Autodesk Inventor part; units mm, degrees
ref_plane "Work Plane1" through (1.525, 0, 0) normal (0, 0, 1) x (1, 0, 0)
ref_plane "YZ Plane" through (0, 0, 0) normal (1, 0, 0) x (0, 1, 0)
ref_plane "XZ Plane" through (0, 0, 0) normal (0, 1, 0) x (-1, 0, 0)
sketch "Sketch1" plane through (0, 0, 0) normal (0, 0, 1) x (1, 0, 0)
  line L0 (0, 4) -> (0, 2.5)
  line L1 (2.4, 2.5) -> (10, 2.5)
  line L2 (10, 2.5) -> (10, 0)
  line L3 (10, 0) -> (-0.5001, 0)
  line L4 (-2.6001, 0) -> (12.1, 0)
  line L5 (-0.5001, 0) -> (-0.5001, 4)
  line L6 (-0.5001, 4) -> (0, 4)
  line L7 (2.4, 2.5) -> (1.9091, 2.5)
  line L8 (1.9091, 2.5) -> (0, 2.5)
  line L9 (0, -0.8) -> (0, 4.8)
  dimension "d0" = 10
  dimension "d1" = 7.6
  dimension "d2" = 5
  dimension "d9" = 0.5001
  dimension "d10" = 8
  dimension "d13" = 0.4909
  dimension "d14" = 5
revolve "Body" add sketch "Sketch1" angle 360 about axis through (10, 0, 0) along (-1, 0, 0)
sketch "Sketch2" plane through (-0.5001, 0, 0) normal (-1, 0, 0) x (0, 0, 1)
  line L0 (0, 4.6188) -> (4, 2.3094)
  line L1 (4, 2.3094) -> (4, -2.3094)
  line L2 (4, -2.3094) -> (0, -4.6188)
  line L3 (0, -4.6188) -> (-4, -2.3094)
  line L4 (-4, -2.3094) -> (-4, 2.3094)
  line L5 (-4, 2.3094) -> (0, 4.6188)
  point P0 (0, 0)
  point P1 (0, 0)
  dimension "d11" = 8
extrude "Head" add sketch "Sketch2" along normal blind 3
sketch "Sketch4" plane through (0, 0, 0) normal (0, 0, 1) x (1, 0, 0)
  line L0 (-3.5001, 4) -> (-3.5001, 4.6188)
  line L1 (-3.5001, 4.6188) -> (-3.1428, 4.6188)
  line L2 (-3.1428, 4.6188) -> (-3.5001, 4)
  line L3 (-4.1001, 0) -> (0.0999, 0)
  line L4 (-0.5001, 4.6188) -> (-3.5001, 4.6188)
  line L5 (-3.5001, 2.3094) -> (-3.5001, 4.6188)
  dimension "d5" = 30
  dimension "d19" = 8
revolve "Chamfer1" cut sketch "Sketch4" angle 360 about axis through (-10, 0, 0) along (1, 0, 0)
thread "Thread"
chamfer "Chamfer2" distance 0.4908 distance2 0.4909 1 edges at (10, -2.5, 0) measured on face at (10, -0.7379, 0.3873)
ref_plane "Work Plane1" through (1.525, 0, 0) normal (0, 0, 1) x (1, 0, 0)
equation "\"d0\" = NLG"
equation "\"d1\" = GEL"
equation "\"d2\" = GD"
equation "\"d10\" = SD2"
equation "\"d14\" = BDM"
equation "\"d11\" = SW"
equation "\"d3\" = KOH - SD"
equation "\"d5\" = ANG1"
equation "\"d19\" = SW0"
equation "\"d15\" = GEL"
equation "\"d6\" = -0.5 * SPD + 0.5 * GD"
equation "\"NLG\" = 10"
equation "\"GD\" = NND"
equation "\"BDM\" = NND"
equation "\"KOH\" = 3.5"
equation "\"GEL\" = 7.6"
equation "\"SW\" = 8"
equation "\"SW0\" = SW"
equation "\"SPD\" = NND - 1.2269 * PTC"
equation "\"SD2\" = SW"
equation "\"SD\" = 0.5"
equation "\"ANG1\" = 30deg"
equation "\"GAL\" = 0.61345 * PTC"
equation "\"GUL\" = 0.61345 * PTC"
equation "\"RR\" = 0.2"
equation "\"WFT\" = SD"
equation "\"GD1\" = THREADDIA - 1.2269 * PTC"
equation "\"THREADDIA\" = 5"
equation "\"SDH\" = SW"
equation "\"TOA\" = 30deg"
equation "\"FAWI\" = 45deg"
equation "\"PTC\" = 0.8"
equation "\"NND\" = 5"
equation "\"E0\" = 1.155 * SW"
properties part number "AS 1110 - M5 x 10" material "Steel, Mild"
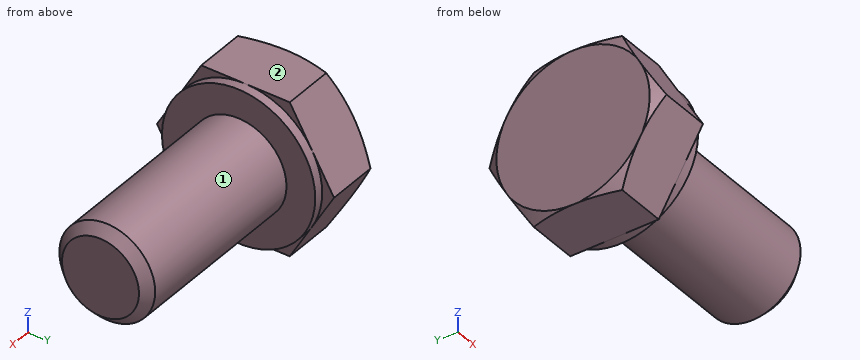
Can you work these out from the model? Positions are in its coordinate system, mm. Face numbers are marked on the shaded views. A direction names the side the tool comes from. Round coordinates to 2 decimals unless told otherwise and drop trailing zeros. Write each loop counter-clockwise with the first axis right and the second up, starting at its lowest first coordinate (ties: lowest second). Pieces come first, ordered by that corner, then holes. Notation, with made-up numbers: (52, 10.25) -> (101, 10.25) arc R22 cw to (101, 32.25) -> close; hole circle Ø2 at (-38, 29). An arc over 180 degrees is marked (long way). Use one line per item in the form item = value. Start each with the question number.
Q1. If I drill on probe 1 along X at (y, z) = (-0.5, 2.75); probe 2 along Z at (x, y) = (8.5, 1.5); probe 3 along Y at (x, z) = (1.25, -0.5), over which ranges is the centre line in solid material (lowest first)? Write a range as [from, to].
Q2. I'm going to push flat-ended pins straight in: P1, Ø1.5, axis at y = -2, z = 1, coming from the +X side; P2, Ø1, axis at y = 1.5, z = -3.5, coming from the +X side; P3, Ø4, axis at x = 5, z = -0.5, coming from the -Y side; P4, Ø2, axis at x = 2, z = 0.5, coming from the +Y side. Where does each tip first touch, or does it pass through?
Q3. Imagine slicing it at A-A (x = -1). Please give me the cut outline in (y, z).
Q4. Which directions (+Z, -Z, +X, -X, +Y, -Y) give clear straight access to the entire face, cutting with the end or side of a thin tool? Please do the marked faces 1 and 2.
Q5. Imagine slicing it at B-B (x = 5.5). Please give me the cut outline in (y, z), then the cut area to 3 significant figures.
Worked out:
q1.probe_1 = [-3.5, 0]
q1.probe_2 = [-2, 2]
q1.probe_3 = [-2.45, 2.45]
q2.P1 = 10
q2.P2 = 0
q2.P3 = -2.5
q2.P4 = 2.5
q3.outline = (-4.62, 0) -> (-2.31, -4) -> (2.31, -4) -> (4.62, 0) -> (2.31, 4) -> (-2.31, 4) -> close
q4.face_1 = +X
q4.face_2 = +Z, +X, -X, +Y, -Y
q5.outline = circle Ø5 at (0, 0)
q5.area = 19.6 mm^2
